Geometry: final body of the model. Coordinates: model frame, mm. A direction names the side the tool comes from. Give positions to 0.01 mm unless a question says otherwise; leave off trailing zeros. Write each loop counter-clockwise with the first axis right and the second up, starting at its lowest first coordinate (ties: lowest second). Pieces come first, ordered by that corner, then holes.
Autodesk Inventor part; units mm, degrees
ref_plane "YZ Plane" through (0, 0, 0) normal (1, 0, 0) x (0, 1, 0)
ref_plane "XZ Plane" through (0, 0, 0) normal (0, 1, 0) x (-1, 0, 0)
ref_plane "XY Plane" through (0, 0, 0) normal (0, 0, 1) x (1, 0, 0)
sketch "Sketch1" plane through (0, 0, 0) normal (1, 0, 0) x (0, 1, 0)
  circle A0 centre (0, 0) radius 4
  dimension "d0" = 8
extrude "Extrusion1" add sketch "Sketch1" along normal blind 1.5
sketch "Sketch2" plane through (1.5, 0, 0) normal (1, 0, 0) x (0, 0, -1)
  circle A0 centre (0, 0) radius 1.15
  arc A1 (-2.1791, 2.7389) -> (-1.5565, 1.9564) centre (-1.8678, 2.3476) ccw
  arc A2 (1.6939, 1.8387) -> (2.3714, 2.5742) centre (2.0326, 2.2065) ccw
  arc A3 (-1.9044, -1.6196) -> (-2.6662, -2.2675) centre (-2.2853, -1.9435) ccw
  arc A4 (1.5526, -3.1368) -> (1.109, -2.2406) centre (1.3308, -2.6887) ccw
  arc A5 (-1.9044, -1.6196) -> (1.109, -2.2406) centre (0, 0) ccw
  arc A6 (1.6939, 1.8387) -> (-1.5565, 1.9564) centre (0, 0) ccw
  arc A7 (-2.6662, -2.2675) -> (1.5526, -3.1368) centre (0, 0) ccw
  arc A8 (2.3714, 2.5742) -> (-2.1791, 2.7389) centre (0, 0) ccw
  dimension "d5" = 2.3
  dimension "d6" = 1
  dimension "d7" = 1
  dimension "d8" = 1
  dimension "d9" = 1
extrude "Extrusion2" cut sketch "Sketch2" against normal blind 2
fillet "Fillet1" radius 0.2 1 edges at (1.5, -4, 0)
fillet "Fillet2" radius 0.2 1 edges at (0, -4, 0)
sketch "Sketch6" plane through (1.5, 0, 0) normal (1, 0, 0) x (0, 0, -1)
  circle A0 centre (2.1297, -1.0387) radius 0.3
  point P0 (0, 0)
  dimension "d20" = 0.6
extrude "Extrusion5" add sketch "Sketch6" along normal blind 2.5
sketch "Sketch7" plane through (0, 0, 0) normal (-1, 0, 0) x (0, 0, 1)
  point P0 (0, 0)
properties part number "compression wheel"
Q1. Ray query, line 1 along Y through (x, z) = (1.2, -0.5); line 2 along X through (y, z) = (-1.5, 1.25); line 3 along Y through (x, z) = (1.35, -1.5). Return the intervals inside material, ascending.
Filled sheet:
line 1: y = -3.97 to -3.46, -2.45 to -1.04, 1.04 to 2.45, 3.46 to 3.97
line 2: x = 0 to 1.5
line 3: y = -3.7 to -3.16, -2.22 to 2, 3.16 to 3.7
Q2. Pin query (flat end, axial travel): P1, Ø3, axis at y = -0.5, z = 3, coming from the -X side; P2, Ø2, axis at x = 2, y = -1.5, coming from the +Z side; P3, Ø2, axis at y = 0, z = 0, coming from the -X side. Return the tip coordinate at first contact, or that it passes through.
Filled sheet:
P1: stops at x = 0
P2: stops at z = 3.93
P3: passes through
Q3. Pull-direction query (Z, two-part tool) for faces 3 (the cylindrical face through (0.76, -1.556, 2.601)), 4 (the cylindrical face through (0.742, -0.867, 3.905)), 5 (the flat face through (1.5, -1, -1)); classes: released by +Z, released by -Z, zero draft, split by the parting line, or undercut.
Filled sheet:
face 3: undercut
face 4: split by the parting line
face 5: zero draft
Q4. Section C-C on x = 0.3. Output: boundary loops of the cut face in (y, z), plus the area to 3 significant figures.
Filled sheet:
outline: circle Ø8 at (0, 0); hole (-3.14, -1.55) arc R0.5 ccw to (-2.24, -1.11) arc R2.5 cw to (-1.62, 1.9) arc R0.5 ccw to (-2.27, 2.67) arc R3.5 ccw to start; hole circle Ø2.3 at (0, 0); hole (1.84, -1.69) arc R0.5 ccw to (2.57, -2.37) arc R3.5 ccw to (2.74, 2.18) arc R0.5 ccw to (1.96, 1.56) arc R2.5 cw to start
area: 36.3 mm2
Q5. Section B-B on y = 0. Output: boundary loops of the cut face in (x, z).
Filled sheet:
outline: (0, -3.8) arc R0.2 ccw to (0.2, -4) - (1.3, -4) arc R0.2 ccw to (1.5, -3.8) - (1.5, -1.15) - (0, -1.15) - close; (0, 1.15) - (1.5, 1.15) - (1.5, 3.8) arc R0.2 ccw to (1.3, 4) - (0.2, 4) arc R0.2 ccw to (0, 3.8) - close
Q6. Access query for faces 1 (the cylindrical face through (0.76, 3.496, -0.161)), 2 (the flat face through (0, -1, -1)). Directions: +Z, -Z, +X, -X, +Y, -Y. A direction counts if a zero-diameter tool reaches every point of the face in a straight line with its end or side. Return the directions, or none.
Filled sheet:
face 1: +X, -X
face 2: +Z, -Z, -X, +Y, -Y
Q7. Section A-A on z = 0. Output: boundary loops of the cut face in (x, y), plus the area to 3 significant figures.
Filled sheet:
outline: (0, -3.8) arc R0.2 ccw to (0.2, -4) - (1.3, -4) arc R0.2 ccw to (1.5, -3.8) - (1.5, -3.5) - (0, -3.5) - close; (0, -2.5) - (1.5, -2.5) - (1.5, -1.15) - (0, -1.15) - close; (0, 1.15) - (1.5, 1.15) - (1.5, 2.5) - (0, 2.5) - close; (0, 3.5) - (1.5, 3.5) - (1.5, 3.8) arc R0.2 ccw to (1.3, 4) - (0.2, 4) arc R0.2 ccw to (0, 3.8) - close
area: 5.52 mm2
Q8. Section D-D on x = 1.75. Output: boundary loops of the cut face in (y, z), plus the area to 3 significant figures.
Filled sheet:
outline: circle Ø0.6 at (-1.04, -2.13)
area: 0.283 mm2
